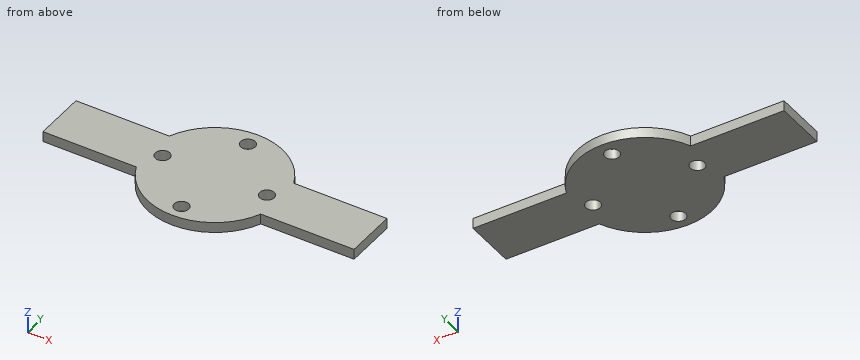
```python
from build123d import *

# Parameters (mm, degrees)
SKIZZE1_R                       = 32.5
AUFSATZ_LINEAR_AUSTRAGEN1_DEPTH = 5
SKIZZE2_R                       = 3.5
SCHNITT_LINEAR_AUSTRAGEN1_DEPTH = 10
SKIZZE3_W                       = 150
SKIZZE3_H                       = 25
AUFSATZ_LINEAR_AUSTRAGEN2_DEPTH = 5
KREISMUSTER1_COUNT              = 4


with BuildPart() as part:
    # Skizze1 → Aufsatz-Linear austragen1 (new body)
    with BuildSketch(Plane.XY):
        Circle(SKIZZE1_R)
    extrude(amount=AUFSATZ_LINEAR_AUSTRAGEN1_DEPTH)

    # Skizze2 → Schnitt-Linear austragen1 (cut)
    with BuildSketch(Plane(origin=(0, 0, 0), x_dir=(-1, 0, 0), z_dir=(0, 0, -1))):
        with Locations((0, 25)):
            Circle(SKIZZE2_R)
    schnitt_linear_austragen1 = extrude(amount=-SCHNITT_LINEAR_AUSTRAGEN1_DEPTH, mode=Mode.SUBTRACT)

    # Skizze3 → Aufsatz-Linear austragen2 (add)
    with BuildSketch(Plane(origin=(0, 0, 0), x_dir=(-1, 0, 0), z_dir=(0, 0, -1))):
        Rectangle(SKIZZE3_W, SKIZZE3_H)
    extrude(amount=-AUFSATZ_LINEAR_AUSTRAGEN2_DEPTH)

    # Kreismuster1: Schnitt-Linear austragen1 ×4 about axis
    kreismuster1_axis = Axis((0, -0.17666974, 0), (0, 0, 1))
    for i in range(1, KREISMUSTER1_COUNT):
        add(schnitt_linear_austragen1.rotate(kreismuster1_axis, i * 360 / KREISMUSTER1_COUNT), mode=Mode.SUBTRACT)


solid = part.part
```
Work out the finished part from the listing and answer in its coordinate system (mm). Round coordinates to 2 decimals unless told otherwise and drop trailing zeros. Order: outer loops, then holes, each group sorted by start corner. A loop starts at its lowest first (then second) coordinate and runs counter-clockwise, first axis right, second up.
Q1. A cutting plane is placed at D-D, the plane x = 35.5. Determine the outline of the cut face in (y, z).
Solution:
outline: (-12.5, 0) - (12.5, 0) - (12.5, 5) - (-12.5, 5) - close
Q2. A cutting plane is placed at B-B, the plane z = 1.1. Determine the outline of the cut face in (x, y).
Solution:
outline: (-75, -12.5) - (-30, -12.5) arc R32.5 ccw to (30, -12.5) - (75, -12.5) - (75, 12.5) - (30, 12.5) arc R32.5 ccw to (-30, 12.5) - (-75, 12.5) - close; hole circle Ø7 at (-25.18, -0.18); hole circle Ø7 at (0, -25.35); hole circle Ø7 at (0, 25); hole circle Ø7 at (25.18, -0.18)
Q3. Given pin 1 Ø9 at (x, y) = (-25.18, -0.18) entering from -Z; pin 2 Ø3 at (x, z) = (36.5, 1.5) entering from -Y; pin 3 Ø2 at (y, z) = (-17.5, 4.5) entering from +X; pin 4 Ø2.5 at (x, z) = (51.5, 3) entering from +Y, each flat-ended and moving along its own axis, determine where each tip first touches the part or whether it passes through.
Solution:
pin 1: stops at z = 0
pin 2: stops at y = -12.5
pin 3: stops at x = 28
pin 4: stops at y = 12.5
Q4. A cutting plane is placed at C-C, the plane y = 25. Determine the outline of the cut face in (x, z).
Solution:
outline: (-20.77, 0) - (-3.5, 0) - (-3.5, 5) - (-20.77, 5) - close; (3.5, 0) - (20.77, 0) - (20.77, 5) - (3.5, 5) - close
Q5. A cutting plane is placed at A-A, the plane x = 0. Determine the outline of the cut face in (y, z).
Solution:
outline: (-32.5, 0) - (-28.85, 0) - (-28.85, 5) - (-32.5, 5) - close; (-21.85, 0) - (21.5, 0) - (21.5, 5) - (-21.85, 5) - close; (28.5, 0) - (32.5, 0) - (32.5, 5) - (28.5, 5) - close
Q6. Find the intervals of material crossed by line 1 along Y through (x, z) = (0, 1.45); line 2 along Y through (x, z) = (-53, 2.35); line 3 along Y through (x, z) = (-25, 3.25), in increasing order.
Solution:
line 1: y = -32.5 to -28.85, -21.85 to 21.5, 28.5 to 32.5
line 2: y = -12.5 to 12.5
line 3: y = -20.77 to -3.67, 3.32 to 20.77
